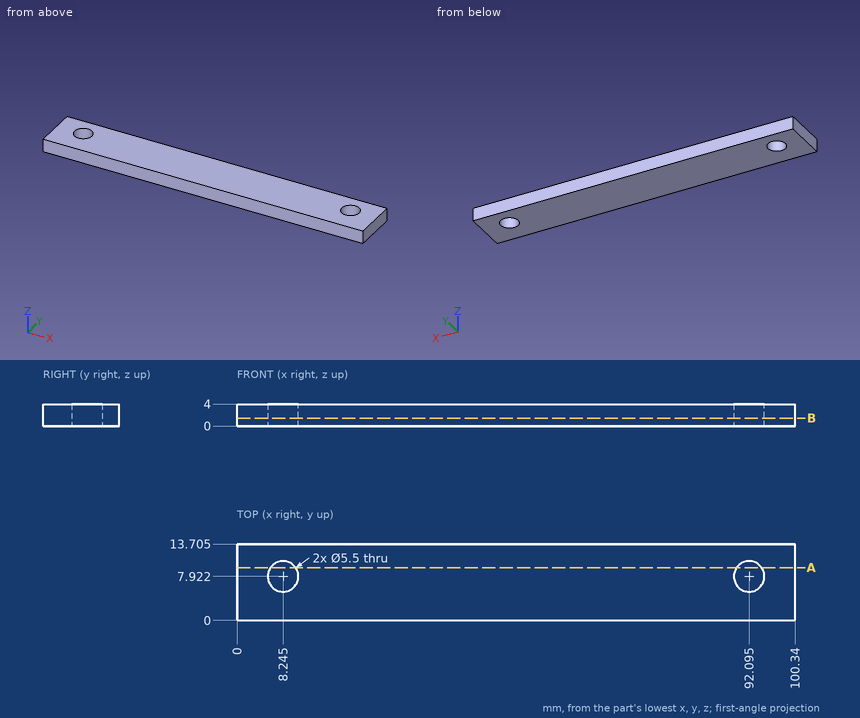
Job drawing, mm, ordinate dimensions from the low corner. One solid piece. Give positions to 0.01 mm unless a question says otherwise; leave off trailing zeros. Write each loop counter-clockwise with the first axis right and the second up, starting at its lowest first coordinate (ties: lowest second). Pieces come first, ordered by that corner, then holes. Notation, with made-up numbers: (66, -18) - (101, -18) arc R18 ccw to (101, -9) - close; hole circle Ø1 at (27.5, 62.25). An arc over 180 degrees is marked (long way). Use one line per item in the form item = value. Start each with the question number.
1. Band-saw the part on A-A on y = 9.5. Write the cut outline in (x, z), plus the area to 3 significant figures.
2. Probe line 1 (X direction, y = 9.25, z = 2); line 2 (X direction, y = 9.75, z = 0.9); line 3 (Y direction, x = 7, z = 2.9) (1 decimal). List the from-to ranges inside material, lowest first. Write a range as [from, to].
3. Band-saw the part on B-B on z = 1.45. Count the separate pieces of the cut face and the enclosed holes in it, plus the area to 3 significant figures.
Conclusion:
q1.outline = (0, 0) - (5.99, 0) - (5.99, 4) - (0, 4) - close; (10.5, 0) - (89.84, 0) - (89.84, 4) - (10.5, 4) - close; (94.35, 0) - (100.34, 0) - (100.34, 4) - (94.35, 4) - close
q1.area = 365 mm²
q2.line_1 = [0, 5.84], [10.65, 89.69], [94.5, 100.34]
q2.line_2 = [0, 6.19], [10.3, 90.04], [94.15, 100.34]
q2.line_3 = [0, 5.5], [10.4, 13.7]
q3.separate_pieces = 1
q3.enclosed_holes = 2
q3.area = 1,330 mm²
